Job drawing, mm, ordinate dimensions from the low corner. One solid piece. A direction names the side the tool comes from. Coordinates: 2 decimals unless noted, no trailing zeros. Loops run counter-clockwise (first coordinate to the right, second up) from the corner with the lowest first, then second, coordinate; pieces in that order, holes last. Notation, with made-up numbers: (-20.5, 59.25) -> (2.5, 59.25) arc R10 ccw to (2.5, 74.25) -> close; hole circle Ø10 at (56.5, 61). An arc over 180 degrees is marked (long way). Answer as CSV lines item,"result". Start each with the question number.
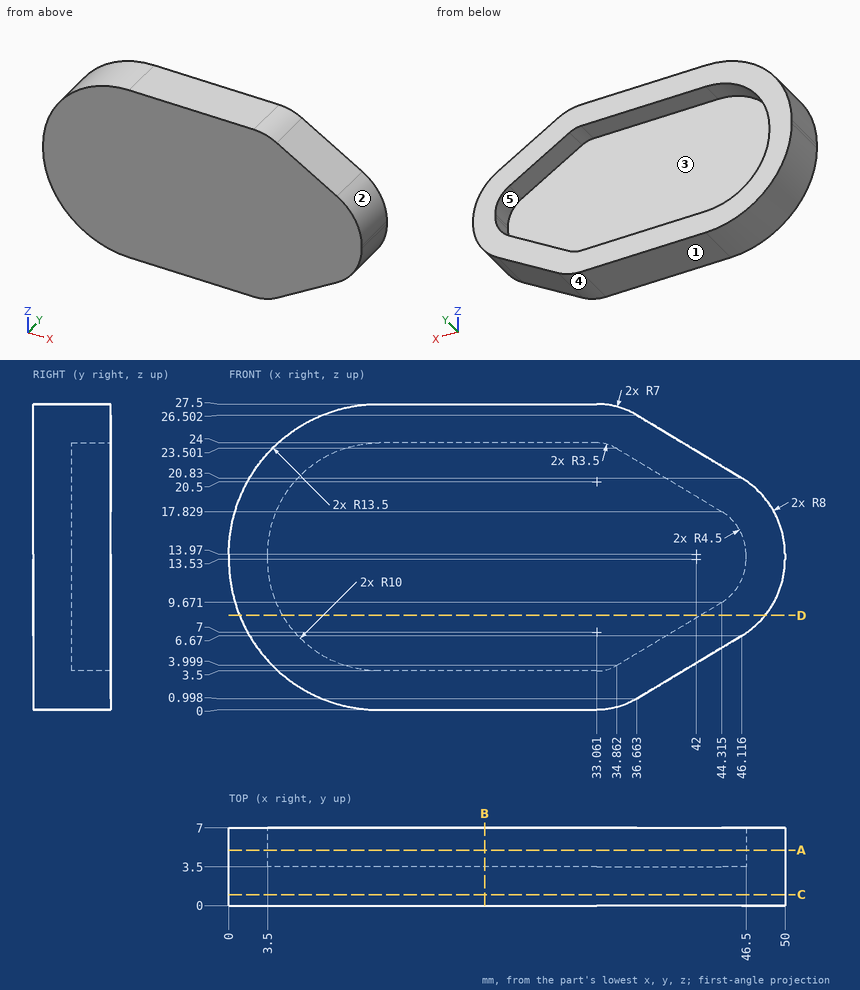
Item 1: Saw through at D-D (z = 8.5). Write the cut outline in (x, y).
Item 2: Flat gauge pins, fed straight in: pin 1 Ø1.5 at (x, z) = (26.5, 3) entering from -Y; pin 2 Ø1 at (y, z) = (5.5, 12.5) entering from +X; pin 3 Ø2 at (x, y) = (5.5, 3) entering from +Z; pin 4 Ø16.5 at (x, z) = (31, 12.5) entering from +Y. Where does each tip first touch, or does it go through?
Item 3: Saw through at B-B (x = 23). Write the cut outline in (y, z).
Item 4: Which spindle directions (+Z, -Z, +X, -X, +Y, -Y) get a long thin tool onto all of the face, cutting with end or side? Do the marked faces 4 and 5. Say none if no direction does.
Item 5: Saw through at A-A (y = 5). Write the cut outline in (x, z) (1 decimal).
Item 6: Saw through at C-C (y = 1). Write the cut outline in (x, z).
Item 7: Two-plate mould, pull along X, no slides. Class the marked faces 1, 2 and 3: pulls with the +X half, pulls with the -X half, needs draft (parallel to the pull), parting line crosses it, or undercut.
Item 8: Wall check: probe 1 along Y at (x, z) = (30.5, 20.5); probe 2 along Z at (x, y) = (14, 3.75); probe 3 along Z at (x, y) = (35, 5) (1 decimal). Give the ranges that are in metal, low to high.
Geometry check:
1,outline,"(0.96, 0) -> (48.22, 0) -> (48.22, 7) -> (42.36, 7) -> (42.36, 3.5) -> (4.84, 3.5) -> (4.84, 7) -> (0.96, 7) -> close"
2,pin 1,"y = 0"
2,pin 2,"x = 49.98"
2,pin 3,"z = 25.54"
2,pin 4,"y = 3.5"
3,outline,"(0, 0) -> (7, 0) -> (7, 3.5) -> (3.5, 3.5) -> (3.5, 24) -> (7, 24) -> (7, 27.5) -> (0, 27.5) -> close"
4,face 4,"-Z, +X, +Y, -Y"
4,face 5,"+Y"
5,outline,"(0, 13.5) arc R13.5 ccw to (13.5, 0) -> (33.1, 0) arc R7 ccw to (36.7, 1) -> (46.1, 6.7) arc R8 ccw to (50, 13.5) -> (50, 14) arc R8 ccw to (46.1, 20.8) -> (36.7, 26.5) arc R7 ccw to (33.1, 27.5) -> (13.5, 27.5) arc R13.5 ccw to (0, 14) -> close; hole (3.5, 13.5) arc R10 ccw to (13.5, 3.5) -> (33.1, 3.5) arc R3.5 ccw to (34.9, 4) -> (44.3, 9.7) arc R4.5 ccw to (46.5, 13.5) -> (46.5, 14) arc R4.5 ccw to (44.3, 17.8) -> (34.9, 23.5) arc R3.5 ccw to (33.1, 24) -> (13.5, 24) arc R10 ccw to (3.5, 14) -> close"
6,outline,"(0, 13.5) arc R13.5 ccw to (13.5, 0) -> (33.06, 0) arc R7 ccw to (36.66, 1) -> (46.12, 6.67) arc R8 ccw to (50, 13.53) -> (50, 13.97) arc R8 ccw to (46.12, 20.83) -> (36.66, 26.5) arc R7 ccw to (33.06, 27.5) -> (13.5, 27.5) arc R13.5 ccw to (0, 14) -> close"
7,face 1,"needs draft"
7,face 2,"pulls with the +X half"
7,face 3,"undercut"
8,probe 1,"0 to 3.5"
8,probe 2,"0 to 3.5, 24 to 27.5"
8,probe 3,"0.3 to 4.1, 23.4 to 27.2"
